```python
from build123d import *

# Parameters (mm, degrees)
F0_W     = 42
F0_H     = 23
F1_DEPTH = 3.2
F2_R     = 6.801578
F3_DEPTH = 6


with BuildPart() as f1:
    # F0 (on Right) → F1 (new body)
    with BuildSketch(Plane.YZ):
        with Locations((-4.014331, 8.529418)):
            Rectangle(F0_W, F0_H)
    extrude(amount=F1_DEPTH)

    # F2 (on Right) → F3 (join)
    with BuildSketch(Plane.YZ):
        with Locations((-14.052913, 9.053115)):
            Circle(F2_R)
        with Locations((6.515576, 9.053115)):
            Circle(F2_R)
    extrude(amount=F3_DEPTH)


solid = f1.part
```
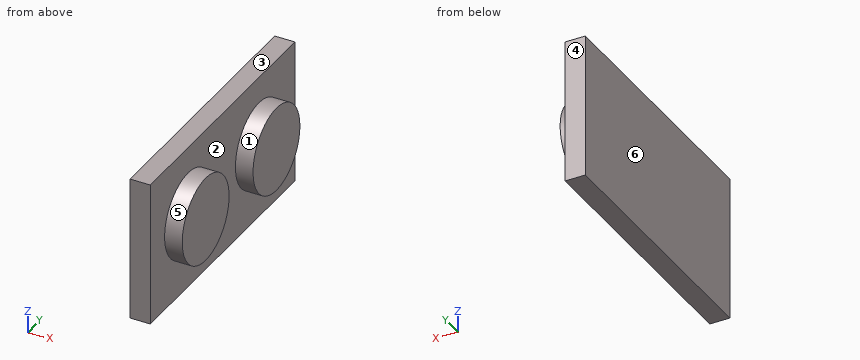
Geometry check sheet. Reference: the model listing, model coordinates, mm. Face numbers are marked on the shaded views. A direction names the side the tool comes from. Round coordinates to 2 decimals unless told otherwise and drop trailing zeros. Order: outer loops, then holes, each group sorted by start corner. A loop starts at its lowest first (then second) coordinate and runs counter-clockwise, first axis right, second up. Notation, with made-up numbers: (67.5, 59) - (112.5, 59) arc R24 ccw to (112.5, 76) - close; hole circle Ø9 at (63, -1). An arc over 180 degrees is marked (long way). Use a Markdown table: item, result. Add a question column.
1) Thickness scan on line 1 along Y through (x, z) = (4.55, 12.75); line 2 along Y through (x, z) = (5.35, 4.75); line 3 along X through (y, z) = (-4, 12.75). Record the ranges inside material, lowest first.
2) Set-up check for the marked faces 5 and 6: record each of +Z, -Z, +X, -X, +Y, -Y from which the full face is reachable in a straight line by a thin tool's end or side.
3) Section check D-D (z = 15). Record the cut outline in (x, y), then the cut area to 3 significant figures.
4) Section check A-A (z = 6.75). Record the cut outline in (x, y).
5) Gauge pin test, flat ends, axial feed: P1, Ø11.5, axis at y = -0.5, z = 5.5, coming from the +X side; P2, Ø1, axis at x = 5, y = -17, coming from the +Z side. Record the tip position at first contact, or that the pin passes through.
6) Mould release check, pull along Y, two halves, no side actions. Record for the marked faces 1, 2, 3 and 4: released by +Y, released by -Y, zero draft, split by the parting line, or undercut.
7) Section check C-C (x = 4.15). Record the cut outline in (y, z).
8) Section check B-B (y = 11.5). Record the cut outline in (x, z), then the cut area to 3 significant figures.
Established:
| question | item | result |
|---|---|---|
| 1 | line 1 | -19.76 to -8.34, 0.81 to 12.22 |
| 1 | line 2 | -19.32 to -8.79, 1.25 to 11.78 |
| 1 | line 3 | 0 to 3.2 |
| 2 | face 5 | +X |
| 2 | face 6 | +Z, -Z, -X, +Y, -Y |
| 3 | outline | (0, -25.01) - (3.2, -25.01) - (3.2, -17.35) - (6, -17.35) - (6, -10.75) - (3.2, -10.75) - (3.2, 3.21) - (6, 3.21) - (6, 9.82) - (3.2, 9.82) - (3.2, 16.99) - (0, 16.99) - close |
| 3 | area | 171 mm2 |
| 4 | outline | (0, -25.01) - (3.2, -25.01) - (3.2, -20.45) - (6, -20.45) - (6, -7.65) - (3.2, -7.65) - (3.2, 0.12) - (6, 0.12) - (6, 12.92) - (3.2, 12.92) - (3.2, 16.99) - (0, 16.99) - close |
| 5 | P1 | x = 6 |
| 5 | P2 | z = 15.4 |
| 6 | face 1 | undercut |
| 6 | face 2 | undercut |
| 6 | face 3 | zero draft |
| 6 | face 4 | released by +Y |
| 7 | outline | circle Ø13.6 at (-14.05, 9.05); circle Ø13.6 at (6.52, 9.05) |
| 8 | outline | (0, -2.97) - (3.2, -2.97) - (3.2, 4.43) - (6, 4.43) - (6, 13.68) - (3.2, 13.68) - (3.2, 20.03) - (0, 20.03) - close |
| 8 | area | 99.5 mm2 |
